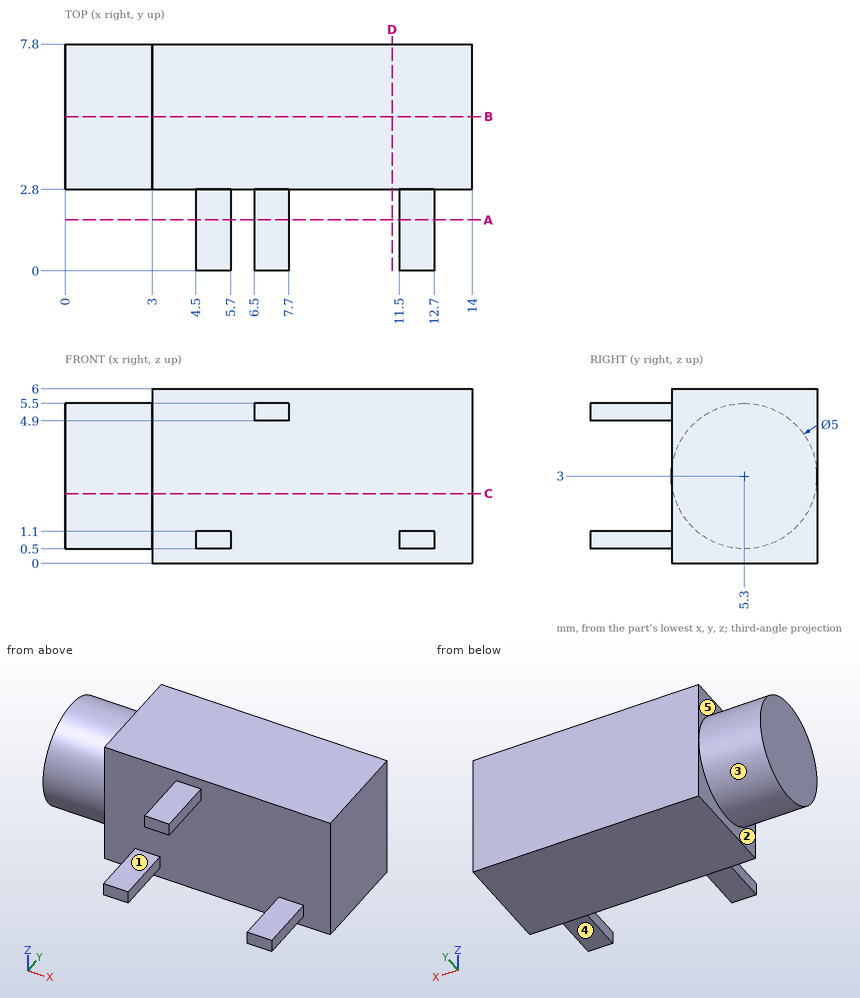
Geometry: see drawing. Coordinates: mm, zero at the bounding-box minimum. A direction names the side the tool comes from. Coordinates: 2 decimals unless noted, no trailing zeros. Write each loop counter-clockwise with the first axis right and the second up, starting at its lowest first coordinate (ties: lowest second). Pieces come first, ordered by that corner, then holes. Notation, with made-up numbers: (28, -27.75) - (84, -27.75) arc R20 ccw to (84, -11.75) - close; hole circle Ø10 at (47, 12.5). An arc over 180 degrees is marked (long way). Put each result on its own line as item: value. Start each with the question number.
1) Cut plane A-A (y = 1.75). Return the cut outline in (x, z).
2) Cut plane D-D (x = 11.25). Return the cut outline in (y, z).
3) Cut plane B-B (y = 5.3). Return the cut outline in (x, z).
4) Contact query for flat-ended pins moving along their axis: pin 1 (1.5 mm diameter, centred on x = 3, z = 2.5, fed in from -Y); pin 2 (1 mm diameter, centred on x = 5, y = 1, fed in from +Z); pin 3 (0.5 mm diameter, centred on y = 1.5, z = 0.5, fed in from -X). Output: stop coordinate, or through.
5) Ray query, L1, parallel to Y at x = 3.5, z = 5.25; L2, parallel to X at y = 3, z = 4.6; L3, parallel to Z at x = 5.25, y = 1.75. Return the intervals inside material, ascending.
6) Cut plane C-C (z = 2.4). Return the cut outline in (x, y).
7) Reachability of the marked faces 1, 2, 3, 4 and 5 from +Z, -Z, +X, -X, +Y, -Y: full face, straight path, thin tool, end or side. Return the list, or none.
Resolved:
1. outline: (4.5, 0.5) - (5.7, 0.5) - (5.7, 1.1) - (4.5, 1.1) - close; (6.5, 4.9) - (7.7, 4.9) - (7.7, 5.5) - (6.5, 5.5) - close; (11.5, 0.5) - (12.7, 0.5) - (12.7, 1.1) - (11.5, 1.1) - close
2. outline: (2.8, 0) - (7.8, 0) - (7.8, 6) - (2.8, 6) - close
3. outline: (0, 0.5) - (3, 0.5) - (3, 0) - (14, 0) - (14, 6) - (3, 6) - (3, 5.5) - (0, 5.5) - close
4. pin 1: stops at y = 2.8
4. pin 2: stops at z = 1.1
4. pin 3: stops at x = 4.5
5. L1: y = 2.8 to 7.8
5. L2: x = 3 to 14
5. L3: z = 0.5 to 1.1
6. outline: (0, 2.87) - (3, 2.87) - (3, 2.8) - (14, 2.8) - (14, 7.8) - (3, 7.8) - (3, 7.73) - (0, 7.73) - close
7. face 1: +Z, +X, -X, -Y
7. face 2: -Z, -X
7. face 3: -X
7. face 4: -Z, +X, -X, -Y
7. face 5: +Z, -X
